```python
from build123d import *

# Parameters (mm, degrees)
BOSS_EXTRUDE1_DEPTH = 12.7
SKETCH7_R           = 1.6
CUT_EXTRUDE2_DEPTH  = 12.7
CIRPATTERN1_COUNT   = 3
CUT_EXTRUDE3_DEPTH  = 11.684
CIRPATTERN2_COUNT   = 3
CUT_EXTRUDE5_DEPTH  = 0.7
FILLET2_R           = 2.54


with BuildPart() as part:
    # Sketch1 → Boss-Extrude1 (new body)
    with BuildSketch(Plane(origin=(0, 0, 0), x_dir=(1, 0, 0), z_dir=(0, 1, 0))):
        Polygon((11.43, -19.797340731), (22.86, 0), (11.43, 19.797340731), (-11.43, 19.797340731), (-22.86, 0), (-11.43, -19.797340731), align=None)
    extrude(amount=BOSS_EXTRUDE1_DEPTH)

    # Sketch5 → Cut-Revolve1 (revolve, cut)
    with BuildSketch(Plane(origin=(0, 12.7, 0), x_dir=(1, 0, 0), z_dir=(0, 1, 0))):
        Polygon((0, -19.797340731), (0, -4.672340739), (-3.81, -4.672340739), (-3.81, -10.797340731), (-11.100000152, -10.797340731), (-11.100000152, -17.797340731), (-6.5, -17.797340731), (-6.5, -19.797340731), align=None)
    cut_revolve1 = revolve(axis=Axis((0, 12.7, 19.797340731), (0, 0, -1)), mode=Mode.SUBTRACT)

    # Sketch7 → Cut-Extrude2 (cut)
    with BuildSketch(Plane(origin=(0, 12.7, 0), x_dir=(1, 0, 0), z_dir=(0, 1, 0))):
        with Locations(Location((0, 10.16, 0), (0, 0, 270))):
            Circle(SKETCH7_R)
        with Locations(Location((8.798818102, -5.08, 0), (0, 0, 270))):
            Circle(SKETCH7_R)
        with Locations(Location((-8.798818102, -5.08, 0), (0, 0, 270))):
            Circle(SKETCH7_R)
    extrude(amount=-CUT_EXTRUDE2_DEPTH, mode=Mode.SUBTRACT)

    # CirPattern1: Cut-Revolve1 ×3 about axis
    cirpattern1_axis = Axis((0, 0, 0), (0, 1, 0))
    for i in range(1, CIRPATTERN1_COUNT):
        add(cut_revolve1.rotate(cirpattern1_axis, i * 360 / CIRPATTERN1_COUNT), mode=Mode.SUBTRACT)

    # Sketch8 → Cut-Extrude3 (cut)
    with BuildSketch(Plane.XY.offset(19.797340731)):
        with BuildLine():
            Line((-13.856406592, 12.7), (-18.662949192, 12.7))
            Line((-18.662949192, 12.7), (-18.662949192, 0))
            Line((-18.662949192, 0), (18.662949192, 0))
            Line((18.662949192, 0), (18.662949192, 12.7))
            Line((18.662949192, 12.7), (13.856406592, 12.7))
            ThreePointArc((13.856406592, 12.7), (0, 0.69999987), (-13.856406592, 12.7))
        make_face()
    cut_extrude3 = extrude(amount=-CUT_EXTRUDE3_DEPTH, mode=Mode.SUBTRACT)

    # CirPattern2: Cut-Extrude3 ×3 about axis
    cirpattern2_axis = Axis((0, 0, 0), (0, 1, 0))
    for i in range(1, CIRPATTERN2_COUNT):
        add(cut_extrude3.rotate(cirpattern2_axis, i * 360 / CIRPATTERN2_COUNT), mode=Mode.SUBTRACT)

    # Sketch10 → Cut-Extrude5 (cut)
    with BuildSketch(Plane.XZ):
        Polygon((14.052718364, 8.113340731), (-14.052718364, 8.113340731), (0, -16.226681461), align=None)
    extrude(amount=-CUT_EXTRUDE5_DEPTH, mode=Mode.SUBTRACT)

    # Fillet2
    # the kernel refuses this fillet: 2.54 mm, written as the material it takes off along each edge
    with BuildSketch(Plane(origin=(14.052718364, -10.298522628, 8.113340731), x_dir=(-0.4999999999999996, 0, -0.8660254037844387), z_dir=(0, 1, 0))) as fillet2_piece_1_section:
        with BuildLine():
            CenterArc((FILLET2_R * 1.73205080757, FILLET2_R), FILLET2_R, 150, 120)
            Line((FILLET2_R * 0.866025403784, FILLET2_R * 1.5), (0, 0))
            Line((0, 0), (FILLET2_R * 1.73205080757, 0))
        make_face()
    fillet2_piece_1 = extrude(amount=33.997045256, mode=Mode.PRIVATE)
    fillet2_piece_1 = fillet2_piece_1 - Plane(origin=(6.277314066, 14.7, -3.624208966), x_dir=(-0.49487165940112743, -0.14285714153061227, -0.8571428573086736), z_dir=(0.8660254037844388, 0, -0.49999999999999983)) * Cylinder(14.00000013, 86, mode=Mode.PRIVATE)
    fillet2_piece_1 = fillet2_piece_1 - Plane(origin=(0, 14.7, 7.248417919), x_dir=(0.9897433188022552, -0.14285714153061224, 0), z_dir=(0, 0, 1)) * Cylinder(14.00000013, 86, mode=Mode.PRIVATE)
    add(fillet2_piece_1, mode=Mode.SUBTRACT)
    with BuildSketch(Plane(origin=(0, -10.298522628, -16.226681461), x_dir=(-0.5000000000000003, 0, 0.8660254037844386), z_dir=(0, 1, 0))) as fillet2_piece_2_section:
        with BuildLine():
            CenterArc((FILLET2_R * 1.73205080757, FILLET2_R), FILLET2_R, 150, 120)
            Line((FILLET2_R * 0.866025403784, FILLET2_R * 1.5), (0, 0))
            Line((0, 0), (FILLET2_R * 1.73205080757, 0))
        make_face()
    fillet2_piece_2 = extrude(amount=33.997045256, mode=Mode.PRIVATE)
    fillet2_piece_2 = fillet2_piece_2 - Plane(origin=(6.277314055, 14.7, -3.62420896), x_dir=(-0.49487165940112743, -0.14285714153061227, -0.8571428573086736), z_dir=(0.8660254037844388, 0, -0.49999999999999983)) * Cylinder(14.00000013, 86, mode=Mode.PRIVATE)
    fillet2_piece_2 = fillet2_piece_2 - Plane(origin=(-6.277314066, 14.7, -3.624208966), x_dir=(-0.4948716594011281, -0.14285714153061227, 0.8571428573086732), z_dir=(-0.8660254037844384, 0, -0.5000000000000004)) * Cylinder(14.00000013, 86, mode=Mode.PRIVATE)
    add(fillet2_piece_2, mode=Mode.SUBTRACT)
    with BuildSketch(Plane(origin=(-14.052718364, 23.698522628, 8.113340731), x_dir=(1, 0, 0), z_dir=(0, -1, 0))) as fillet2_piece_3_section:
        with BuildLine():
            CenterArc((FILLET2_R * 1.73205080757, -FILLET2_R), FILLET2_R, 90, 120)
            Line((FILLET2_R * 0.866025403784, -FILLET2_R * 1.5), (0, 0))
            Line((0, 0), (FILLET2_R * 1.73205080757, 0))
        make_face()
    fillet2_piece_3 = extrude(amount=33.997045256, mode=Mode.PRIVATE)
    fillet2_piece_3 = fillet2_piece_3 - Plane(origin=(0, 14.7, 7.248417932), x_dir=(0.9897433188022552, -0.14285714153061224, 0), z_dir=(0, 0, 1)) * Cylinder(14.00000013, 86, mode=Mode.PRIVATE)
    fillet2_piece_3 = fillet2_piece_3 - Plane(origin=(-6.277314055, 14.7, -3.62420896), x_dir=(-0.4948716594011281, -0.14285714153061227, 0.8571428573086732), z_dir=(-0.8660254037844384, 0, -0.5000000000000004)) * Cylinder(14.00000013, 86, mode=Mode.PRIVATE)
    add(fillet2_piece_3, mode=Mode.SUBTRACT)


solid = part.part
```
Verification items for the finished model (mm, model axes). A direction names the side the tool comes from. Give positions to 0.01 mm unless a question says otherwise; leave off trailing zeros. Write each loop counter-clockwise with the first axis right and the second up, starting at its lowest first coordinate (ties: lowest second). Pieces come first, ordered by that corner, then holes. Notation, with made-up numbers: (15, 53) - (69, 53) arc R33 cw to (69, 86) - close; hole circle Ø11 at (63, 77). An arc over 180 degrees is marked (long way). Put each result on its own line as item: value.
Q1. Mould release check, pull along Z, two halves, no side actions. Record for faces 5 (the face through (0, 5, 19.797)), 6 (the face through (0.2, 1.6, 14.3)), 7 (the face through (10, 10, -19.797)): released by +Z, released by -Z, zero draft, split by the parting line, or undercut.
Result:
face 5: released by +Z
face 6: undercut
face 7: released by -Z
Q2. Section check B-B on z = 6. Count the separate pieces of the cut face and the enclosed holes in it, and give its area (3 significant figures).
Result:
separate pieces: 3
enclosed holes: 0
area: 246 mm2
Q3. Set-up check for faces 1 (the face through (8.87, 6.78, 3.48)), 2 (the face through (-7, 2, 8.113)), 3 (the face through (0.1, 6.2, 18.8)), 4 (the face through (9.43, 7.23, -5.26)): record each of +Z, -Z, +X, -X, +Y, -Y from which the full face is reachable in a straight line by a thin tool's end or side.
Result:
face 1: +Y, -Y
face 2: +Z, -X, -Y
face 3: +Z, +Y
face 4: +Y
Q4. Scan lines: probe 1 along X at (y, z) = (7.25, 5.08); probe 2 along X at (y, z) = (5, -10.16); probe 3 along X at (y, z) = (4, -8.5). Record each from-to range of solid material in increasing order. Write a range as from..to.
Result:
probe 1: -14.91..-10.4, -7.2..7.2, 10.4..14.91
probe 2: -16.99..-14.68, -6.6..-1.6, 1.6..6.6, 14.68..16.99
probe 3: -17.95..-15.64, -7.56..7.56, 15.64..17.95
Q5. Section check A-A on z = 11.5. Record the cut outline in (x, y), and give its area (3 significant figures).
Result:
outline: (-13.86, 12.7) arc R14 ccw to (13.86, 12.7) - (11.1, 12.7) arc R11.1 cw to (-11.1, 12.7) - close
area: 58.5 mm2
Q6. Depth check by flat-ended pin: P1, Ø1, axis at x = 12, z = -6.5, coming from the +Y side; P2, Ø12, axis at x = -17.5, z = -9, coming from the +Y side; P3, Ø1.9, axis at x = -0.5, y = 10.5, coming from the +Z side; P4, Ø6, axis at y = 5, z = 13, coming from the -X side. Enter the tip coordinate at first touch or a pass-through.
Result:
P1: y = 1.63
P2: y = 12.7
P3: z = 4.67
P4: x = -12.29
